from build123d import *

# Parameters (mm, degrees)
SKETCH1_R           = 4
SKETCH1_R_2         = 1.85
BOSS_EXTRUDE1_DEPTH = 3.175


with BuildPart() as part:
    # Sketch1 → Boss-Extrude1 (new body)
    with BuildSketch(Plane.XY):
        with BuildLine():
            ThreePointArc((-36, 0), (0, -36), (36, 0))
            ThreePointArc((36, 0), (0, 36), (-36, 0))
        make_face()
        Circle(SKETCH1_R, mode=Mode.SUBTRACT)
        with Locations((-8, 0)):
            Circle(SKETCH1_R_2, mode=Mode.SUBTRACT)
        with Locations((0, -8)):
            Circle(SKETCH1_R_2, mode=Mode.SUBTRACT)
        with Locations((0, 8)):
            Circle(SKETCH1_R_2, mode=Mode.SUBTRACT)
        with Locations((8, 0)):
            Circle(SKETCH1_R_2, mode=Mode.SUBTRACT)
    extrude(amount=BOSS_EXTRUDE1_DEPTH)


solid = part.part
Read the model definition and answer for the solid it produces. Units are mm, in the model's axes. Round coordinates to 2 decimals unless told otherwise and drop trailing zeros. Write each loop counter-clockwise with the first axis right and the second up, starting at its lowest first coordinate (ties: lowest second). Pieces come first, ordered by that corner, then holes.
1. The part is cut by section C-C, the plane z = 0.8. Determine the outline of the cut face in (x, y).
2. The part is cut by section B-B, the plane y = 8. Determine the outline of the cut face in (x, z) (3 decimals), then the cut area to 3 significant figures.
3. The part is cut by section A-A, the plane y = 0. Determine the outline of the cut face in (x, z) (3 decimals), then the cut area to 3 significant figures.
4. Straight lines are drawn through the part: L1, parallel to Y at x = 0, z = 2; L2, parallel to Y at x = -8, z = 2.15; L3, parallel to Y at x = -2.5, z = 2.8. For each, find the intervals that lie inside material, in ascending order.
5. Determine the mould class of faces 1 (the face through (34.34, 10.81, 1.57)), 2 (the face through (-0.867, -3.905, 1.565)), 3 (the face through (7, -7, 3.175)) for opening direction X: pulls with the +X half, pulls with the -X half, needs draft (parallel to the pull), parting line crosses it, or undercut.
6. Given pin 1 Ø6.5 at (x, y) = (0, 0) entering from -Z; pin 2 Ø1.5 at (y, z) = (-2, 2) entering from +X, each flat-ended and moving along its own axis, determine where each tip first touches the part or whether it passes through.
7. The part is cut by section D-D, the plane x = 1. Determine the outline of the cut face in (y, z) (3 decimals).
Values:
1. outline: circle Ø72 at (0, 0); hole circle Ø3.7 at (-8, 0); hole circle Ø8 at (0, 0); hole circle Ø3.7 at (0, -8); hole circle Ø3.7 at (0, 8); hole circle Ø3.7 at (8, 0)
2. outline: (-35.1, 0) - (-1.85, 0) - (-1.85, 3.175) - (-35.1, 3.175) - close; (1.85, 0) - (35.1, 0) - (35.1, 3.175) - (1.85, 3.175) - close
2. area: 211 mm2
3. outline: (-36, 0) - (-9.85, 0) - (-9.85, 3.175) - (-36, 3.175) - close; (-6.15, 0) - (-4, 0) - (-4, 3.175) - (-6.15, 3.175) - close; (4, 0) - (6.15, 0) - (6.15, 3.175) - (4, 3.175) - close; (9.85, 0) - (36, 0) - (36, 3.175) - (9.85, 3.175) - close
3. area: 180 mm2
4. L1: y = -36 to -9.85, -6.15 to -4, 4 to 6.15, 9.85 to 36
4. L2: y = -35.1 to -1.85, 1.85 to 35.1
4. L3: y = -35.91 to -3.12, 3.12 to 35.91
5. face 1: parting line crosses it
5. face 2: undercut
5. face 3: needs draft
6. pin 1: passes through
6. pin 2: stops at x = 35.98
7. outline: (-35.986, 0) - (-9.556, 0) - (-9.556, 3.175) - (-35.986, 3.175) - close; (-6.444, 0) - (-3.873, 0) - (-3.873, 3.175) - (-6.444, 3.175) - close; (3.873, 0) - (6.444, 0) - (6.444, 3.175) - (3.873, 3.175) - close; (9.556, 0) - (35.986, 0) - (35.986, 3.175) - (9.556, 3.175) - close
